Here's the drawing with two shaded views (mm, measured from the low corner). I have some questions. A direction names the side the tool comes from. Round coordinates to 2 decimals unless told otherwise and drop trailing zeros. Order: outer loops, then holes, each group sorted by start corner. A loop starts at its lowest first (then second) coordinate and runs counter-clockwise, first axis right, second up. Notation, with made-up numbers: (89.25, 49) - (126.25, 49) arc R20 cw to (126.25, 77) - close; hole circle Ø11 at (84, -9.75). An arc over 180 degrees is marked (long way). One line per item, written item: value.
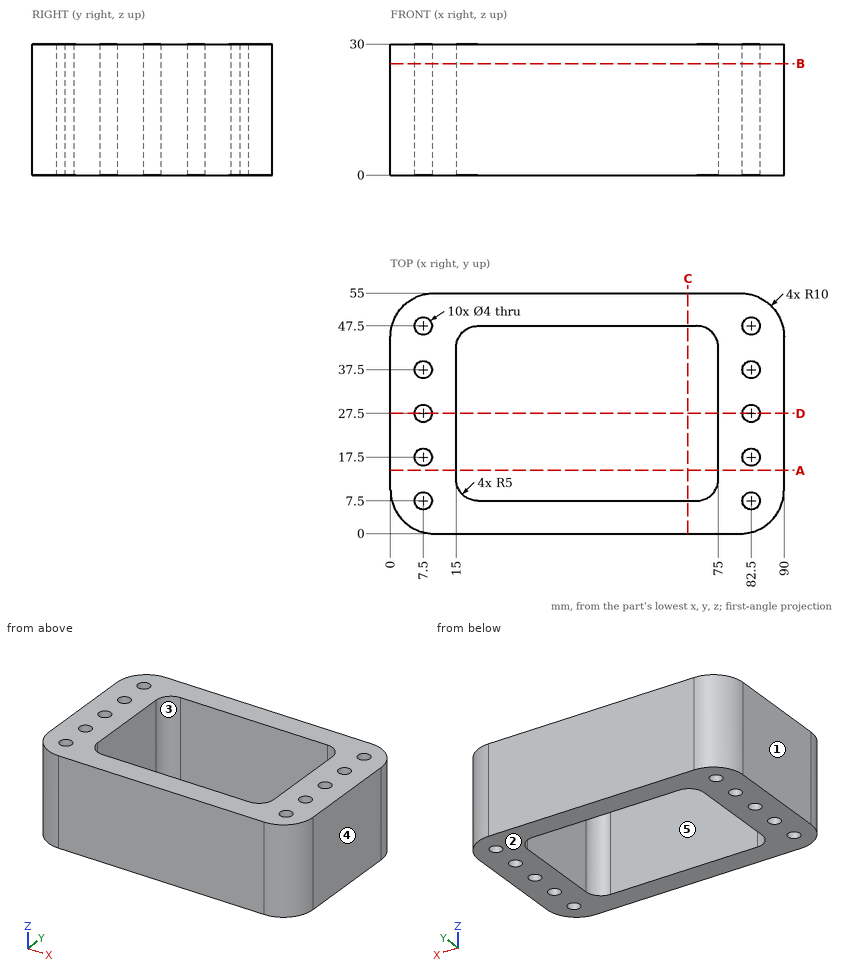
Q1. Will this pin go through, and if not, where does the flat tip stop? pin 1 (12 mm diameter, centred on x = 25.5, y = 33, fed in from +Z).
Results list:
pin 1: through
Q2. We'd pull the mould along X, two halves only. Please class the marked faces 1, 2 and 3: released by +X, released by -X, zero draft, split by the parting line, or undercut.
Results list:
face 1: released by -X
face 2: zero draft
face 3: undercut
Q3. Which directions (+Z, -Z, +X, -X, +Y, -Y) give clear straight access to the entire face, cutting with the end or side of a thin tool? Please do the marked faces 4 and 5.
Results list:
face 4: +Z, -Z, +X, +Y, -Y
face 5: +Z, -Z
Q4. If we section it at B-B, the plane z = 25.5: Give the number of separate pieces and of enclosed holes in the cut face, then the cut area to 3 significant figures.
Results list:
separate pieces: 1
enclosed holes: 11
area: 2,360 mm²
Q5. If I drill on line 1 along X through (y, z) = (22.5, 20.25); line 2 along Y through (x, z) = (42.5, 16); line 3 along X through (y, z) = (18, 15.5), over which ranges is the centre line in solid material (lowest first)?
Results list:
line 1: 0 to 15, 75 to 90
line 2: 0 to 7.5, 47.5 to 55
line 3: 0 to 5.56, 9.44 to 15, 75 to 80.56, 84.44 to 90
Q6. If we section it at A-A, the plane y = 14.5: Please give me the cut outline in (x, z).
Results list:
outline: (0, 0) - (15, 0) - (15, 30) - (0, 30) - close; (75, 0) - (90, 0) - (90, 30) - (75, 30) - close
Q7. If we section it at D-D, the plane y = 27.5: Please give me the cut outline in (x, z), then the cut area to 3 significant figures.
Results list:
outline: (0, 0) - (5.5, 0) - (5.5, 30) - (0, 30) - close; (9.5, 0) - (15, 0) - (15, 30) - (9.5, 30) - close; (75, 0) - (80.5, 0) - (80.5, 30) - (75, 30) - close; (84.5, 0) - (90, 0) - (90, 30) - (84.5, 30) - close
area: 660 mm²
Q8. If we section it at C-C, the plane x = 68: Please give me the cut outline in (y, z), then the cut area to 3 significant figures.
Results list:
outline: (0, 0) - (7.5, 0) - (7.5, 30) - (0, 30) - close; (47.5, 0) - (55, 0) - (55, 30) - (47.5, 30) - close
area: 450 mm²
